The listing builds one solid part. Answer for the finished solid, in the listing's coordinates (mm). Face numbers are marked on the shaded views. A direction names the side the tool comes from. Coordinates: 2 decimals unless noted, no trailing zeros. Order: outer loops, then holes, each group sorted by start corner. A loop starts at its lowest first (then second) coordinate and runs counter-clockwise, first axis right, second up.
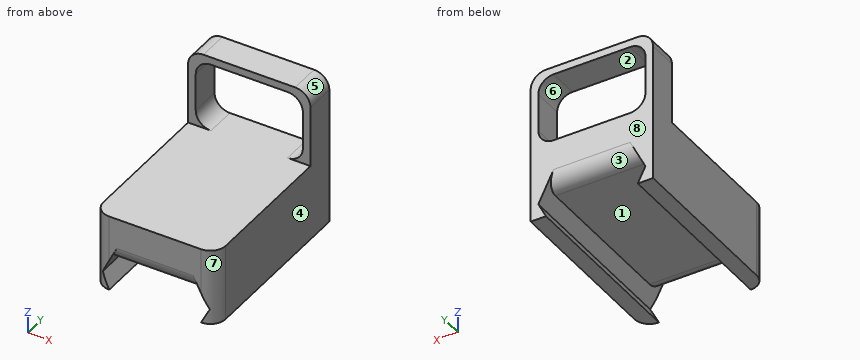
```python
from build123d import *

# Parameters (mm, degrees)
F0_W     = 40
F0_H     = 15
F1_DEPTH = 30
F2_W     = 2.5
F2_H     = 10
F3_DEPTH = 25
F4_W     = 10
F4_H     = 2.5
F5_DEPTH = 35
F6_W     = 5
F6_H     = 60
F7_DEPTH = 10
F9_DEPTH = 60.001
F10_R    = 5


with BuildPart() as f1:
    # F0 (on Front) → F1 (new body, symmetric)
    with BuildSketch(Plane.XZ):
        Rectangle(F0_W, F0_H)
    extrude(amount=F1_DEPTH, both=True)

    # F2 (on face) → F3 (join)
    with BuildSketch(Plane.XY.offset(7.5)):
        with Locations((-18.75, 25)):
            Rectangle(F2_W, F2_H)
        with Locations((18.75, 25)):
            Rectangle(F2_W, F2_H)
    extrude(amount=F3_DEPTH)

    # F4 (on face) → F5 (join, through all)
    with BuildSketch(Plane(origin=(17.5, 0, 0), x_dir=(0, -1, 0), z_dir=(-1, 0, 0))):
        with Locations((-25, 31.25)):
            Rectangle(F4_W, F4_H)
    extrude(amount=F5_DEPTH)

    # F6 (on face) → F7 (join)
    with BuildSketch(Plane(origin=(0, 0, -7.5), x_dir=(1, 0, 0), z_dir=(0, 0, -1))):
        with Locations((-17.5, 0)):
            Rectangle(F6_W, F6_H)
        with Locations((17.5, 0)):
            Rectangle(F6_W, F6_H)
    extrude(amount=F7_DEPTH)

    # F8 (on face) → F9 (cut, through all)
    with BuildSketch(Plane.XZ.offset(30)):
        Polygon((-15, -7.5), (-17.5, -12.5), (-15, -17.5), align=None)
        Polygon((17.5, -12.5), (15, -7.5), (15, -17.5), align=None)
    extrude(amount=-F9_DEPTH, mode=Mode.SUBTRACT)

    # F10
    f10_edges = [f1.edges().sort_by_distance(p)[0] for p in [
        (20, 25, 32.5),
        (-20, 25, 32.5),
        (-17.5, 25, 30),
        (17.5, 25, 30),
        (17.5, 25, 7.5),
        (-17.5, 25, 7.5),
        (20, -30, -5),
        (-20, -30, -5),
        (0, -30, -7.5),
        (0, 30, -7.5),
    ]]
    fillet(f10_edges, radius=F10_R)


solid = f1.part
```
1) A cutting plane is placed at D-D, the plane y = -5. Write down the section's boundary in (x, z), plus the area to 3 significant figures.
2) Each of these flat-tipped pins is pushed along its axis until it touches: P1, Ø6, axis at x = 1, y = -21.5, coming from the -Z side; P2, Ø4, axis at x = -13.5, y = -16.5, coming from the +Z side. Where does it stop, or does it pass through?
3) A cutting plane is placed at A-A, the plane x = 8.5. Write down the section's boundary in (y, z).
4) A cutting plane is placed at C-C, the plane z = 29. Write down the section's boundary in (x, y), plus the area to 3 significant figures.
5) For the marked faces 1, 2, 3, 4 and 5, determine the directions among +Z, -Z, +X, -X, +Y, -Y from which every point of the face is accessible in a straight line to the end or side of a thin tool.
6) Straight lines are drawn through the part: probe 1 along Z at (x, y) = (1.5, -11.5); probe 2 along Y at (x, z) = (-6, 30.5); probe 3 along X at (y, z) = (5.5, -9). For each, find the intervals that lie inside material, in ascending order.
7) A cutting plane is placed at B-B, the plane y = 22.5. Write down the section's boundary in (x, z).
8) The mould has two halves that part along X. Classify the marked faces 6, 7 and 8: released by +X, released by -X, zero draft, split by the parting line, or undercut.
Working result:
1. outline: (-20, -17.5) - (-15, -17.5) - (-17.5, -12.5) - (-15, -7.5) - (15, -7.5) - (17.5, -12.5) - (15, -17.5) - (20, -17.5) - (20, 7.5) - (-20, 7.5) - close
1. area: 675 mm2
2. P1: stops at z = -7.5
2. P2: stops at z = 7.5
3. outline: (-30, -2.5) arc R5 ccw to (-25, -7.5) - (25, -7.5) arc R5 ccw to (30, -2.5) - (30, 7.5) - (-30, 7.5) - close; (20, 30) - (30, 30) - (30, 32.5) - (20, 32.5) - close
4. outline: (-19.77, 20) - (-15.5, 20) - (-15.5, 30) - (-19.77, 30) - close; (15.5, 20) - (19.77, 20) - (19.77, 30) - (15.5, 30) - close
4. area: 85.4 mm2
5. face 1: -Z, +Y, -Y
5. face 2: +Y, -Y
5. face 3: -Z, +Y
5. face 4: +Z, -Z, +X, +Y, -Y
5. face 5: +Z, +X, +Y, -Y
6. probe 1: z = -7.5 to 7.5
6. probe 2: y = 20 to 30
6. probe 3: x = -20 to -15.75, 15.75 to 20
7. outline: (-20, -17.5) - (-15, -17.5) - (-17.5, -12.5) - (-15, -7.5) - (15, -7.5) - (17.5, -12.5) - (15, -17.5) - (20, -17.5) - (20, 27.5) arc R5 ccw to (15, 32.5) - (-15, 32.5) arc R5 ccw to (-20, 27.5) - close; hole (-17.5, 12.5) arc R5 ccw to (-12.5, 7.5) - (12.5, 7.5) arc R5 ccw to (17.5, 12.5) - (17.5, 25) arc R5 ccw to (12.5, 30) - (-12.5, 30) arc R5 ccw to (-17.5, 25) - close
8. face 6: undercut
8. face 7: released by +X
8. face 8: zero draft
